from build123d import *

# Parameters (mm, degrees)
SKETCH1_W           = 76.2
SKETCH1_H           = 38.1
SKETCH1_W_2         = 28
SKETCH1_H_2         = 28
SKETCH1_R           = 3.75
BOSS_EXTRUDE1_DEPTH = 9.525


with BuildPart() as part:
    # Sketch1 → Boss-Extrude1 (new body)
    with BuildSketch(Plane.XY):
        with Locations((38.1, -19.05)):
            Rectangle(SKETCH1_W, SKETCH1_H)
        with Locations((38.1, -19.05)):
            Rectangle(SKETCH1_W_2, SKETCH1_H_2, mode=Mode.SUBTRACT)
        with Locations((38.1, -19.05)):
            Rectangle(SKETCH1_W_2, SKETCH1_H_2)
        with Locations((38.1, -19.05)):
            Circle(SKETCH1_R, mode=Mode.SUBTRACT)
    extrude(amount=BOSS_EXTRUDE1_DEPTH)


solid = part.part
For this review, take the finished solid that the model builds, in its own axes (mm). Coordinates: 2 decimals unless noted, no trailing zeros. Loops run counter-clockwise (first coordinate to the right, second up) from the corner with the lowest first, then second, coordinate; pieces in that order, holes last. Notation, with made-up numbers: (56.25, 7.25) - (63.25, 7.25) arc R23 ccw to (63.25, 38.25) - close; hole circle Ø9 at (8.25, 64). An arc over 180 degrees is marked (long way). Use a Markdown table: item, result. Add a question column.
Item 1: Mouldability with a two-part tool opening along X and no side actions: class faces 1 (the face through (76.2, -19, 5)), 2 (the face through (38, 0, 5)), 3 (the face through (34.354, -18.885, 4.696)), 4 (the face through (0, -19, 5)) as pulls with the +X half, pulls with the -X half, needs draft (parallel to the pull), parting line crosses it, or undercut.
Item 2: For line 1 (Y direction, x = 38.1, z = 7); line 2 (Y direction, x = 41, z = 0.75); line 3 (X direction, y = -20.5, z = 3), list the stretches that pass through material, from the lowest coordinate up.
Item 3: We need section C-C (z = 2.75). Give the boundary of the cut face in (x, y), and give its area (3 significant figures).
Item 4: Insertion check: pin 1 Ø2 at (x, z) = (55, 7) entering from +Y; pin 2 Ø7 at (x, y) = (38.1, -19.05) entering from -Z. Each pin has a flat end and moves straight along its axis. Give the tip position at first contact, or say it passes through.
Item 5: We need section B-B (x = 38.1). Give the boundary of the cut face in (y, z) (3 decimals).
Item 6: We need section A-A (y = -19.05). Give the boundary of the cut face in (x, z) (3 decimals), and give its area (3 significant figures).
Results list:
| question | item | result |
|---|---|---|
| 1 | face 1 | pulls with the +X half |
| 1 | face 2 | needs draft |
| 1 | face 3 | undercut |
| 1 | face 4 | pulls with the -X half |
| 2 | line 1 | y = -38.1 to -22.8, -15.3 to 0 |
| 2 | line 2 | y = -38.1 to -21.43, -16.67 to 0 |
| 2 | line 3 | x = 0 to 34.64, 41.56 to 76.2 |
| 3 | outline | (0, -38.1) - (76.2, -38.1) - (76.2, 0) - (0, 0) - close; hole circle Ø7.5 at (38.1, -19.05) |
| 3 | area | 2,860 mm^2 |
| 4 | pin 1 | stops at y = 0 |
| 4 | pin 2 | passes through |
| 5 | outline | (-38.1, 0) - (-22.8, 0) - (-22.8, 9.525) - (-38.1, 9.525) - close; (-15.3, 0) - (0, 0) - (0, 9.525) - (-15.3, 9.525) - close |
| 6 | outline | (0, 0) - (34.35, 0) - (34.35, 9.525) - (0, 9.525) - close; (41.85, 0) - (76.2, 0) - (76.2, 9.525) - (41.85, 9.525) - close |
| 6 | area | 654 mm^2 |
